Part model, mm, in its own coordinate system. Give positions to 0.01 mm unless a question says otherwise; leave off trailing zeros. Order: outer loops, then holes, each group sorted by start corner. A loop starts at its lowest first (then second) coordinate and runs counter-clockwise, first axis right, second up. Notation, with made-up numbers: (-26.5, 34) - (-9.5, 34) arc R22 ccw to (-9.5, 46) - close; hole circle Ø6 at (41, -20.5). An arc over 180 degrees is marked (long way). Use a Markdown table: item, result. Add a question column.
from build123d import *

# Parameters (mm, degrees)
F1_DEPTH = 3.81
F2_W     = 36.83
F2_H     = 76.2
F3_DEPTH = 3.81


with BuildPart() as f1:
    # F0 (on Top) → F1 (new body)
    with BuildSketch(Plane.XY):
        Polygon((39.453842, -95.25), (95.25, -39.453842), (95.25, 39.453842), (39.453842, 95.25), (-39.453842, 95.25), (-95.25, 39.453842), (-95.25, -39.453842), (-39.453842, -95.25), align=None)
    extrude(amount=F1_DEPTH)

    # F2 (on face) → F3 (cut)
    with BuildSketch(Plane.XY.offset(3.81)):
        with Locations((-63.5, 0)):
            Rectangle(F2_W, F2_H)
    extrude(amount=-F3_DEPTH, mode=Mode.SUBTRACT)

    # F4: F1 across plane


with BuildPart() as f1_1:
    add(f1.part)
    add(f1.part.mirror(Plane.YZ), mode=Mode.INTERSECT)


solid = f1_1.part
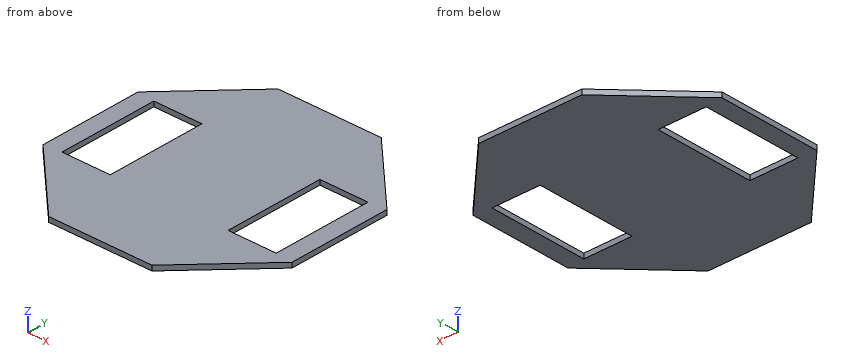
1. Cut at D-D (x = 78). Write the cut outline in (y, z).
2. Cut at B-B (z = 2.5). Write the cut outline in (x, y) (3 decimals), plus the area to 3 significant figures.
3. Pin check, flat tips, straight feed: P1, Ø1.1, axis at x = 62, z = 2, coming from the -Y side; P2, Ø1.5, axis at y = 61.5, z = 2, coming from the -X side. Stop position of each tip, or through.
4. Cut at A-A (y = 22.5). Write the cut outline in (x, z) (3 decimals), plus the area to 3 significant figures.
5. Drill centre lines: probe 1 along X at (y, z) = (35, 2.2) (3 decimals); probe 2 along Y at (x, z) = (-49, 1.45); probe 3 along Y at (x, z) = (63, 1.7). Where is each one in solid material? Low to high. Write a range as [from, to].
6. Cut at C-C (x = -64). Write the cut outline in (y, z), plus the area to 3 significant figures.
Responses:
| question | item | result |
|---|---|---|
| 1 | outline | (-56.7, 0) - (-38.1, 0) - (-38.1, 3.81) - (-56.7, 3.81) - close; (38.1, 0) - (56.7, 0) - (56.7, 3.81) - (38.1, 3.81) - close |
| 2 | outline | (-95.25, -39.454) - (-39.454, -95.25) - (39.454, -95.25) - (95.25, -39.454) - (95.25, 39.454) - (39.454, 95.25) - (-39.454, 95.25) - (-95.25, 39.454) - close; hole (-81.915, -38.1) - (-45.085, -38.1) - (-45.085, 38.1) - (-81.915, 38.1) - close; hole (45.085, -38.1) - (81.915, -38.1) - (81.915, 38.1) - (45.085, 38.1) - close |
| 2 | area | 24,500 mm² |
| 3 | P1 | stops at y = -73.25 |
| 3 | P2 | stops at x = -73.95 |
| 4 | outline | (-95.25, 0) - (-81.915, 0) - (-81.915, 3.81) - (-95.25, 3.81) - close; (-45.085, 0) - (45.085, 0) - (45.085, 3.81) - (-45.085, 3.81) - close; (81.915, 0) - (95.25, 0) - (95.25, 3.81) - (81.915, 3.81) - close |
| 4 | area | 445 mm² |
| 5 | probe 1 | x = [-95.25, -81.915], [-45.085, 45.085], [81.915, 95.25] |
| 5 | probe 2 | y = [-85.7, -38.1], [38.1, 85.7] |
| 5 | probe 3 | y = [-71.7, -38.1], [38.1, 71.7] |
| 6 | outline | (-70.7, 0) - (-38.1, 0) - (-38.1, 3.81) - (-70.7, 3.81) - close; (38.1, 0) - (70.7, 0) - (70.7, 3.81) - (38.1, 3.81) - close |
| 6 | area | 248 mm² |
